Work out the finished part from the listing and answer in its coordinate system (mm). A direction names the side the tool comes from. Coordinates: 2 decimals unless noted, no trailing zeros. Loops run counter-clockwise (first coordinate to the right, second up) from the corner with the lowest first, then second, coordinate; pieces in that order, holes last. Notation, with made-up numbers: (18.25, 49) -> (46.25, 49) arc R38 ccw to (46.25, 88) -> close; hole circle Ø1 at (27, 20.5). An arc over 180 degrees is marked (long way). Use a Markdown table: item, result.
from build123d import *

# Parameters (mm, degrees)
SKETCH2_W           = 25
SKETCH2_H           = 25
BOSS_EXTRUDE1_DEPTH = 25
SKETCH3_R           = 3.25
CUT_EXTRUDE1_DEPTH  = 44.301270189
SKETCH4_R           = 3.25
CUT_EXTRUDE2_DEPTH  = 44.301270189
SKETCH5_R           = 3.25
CUT_EXTRUDE3_DEPTH  = 44.301270189
SKETCH6_R           = 5
CUT_EXTRUDE4_DEPTH  = 23
SKETCH7_R           = 5
CUT_EXTRUDE5_DEPTH  = 23
SKETCH12_R          = 5
CUT_EXTRUDE9_DEPTH  = 23
BOSS_EXTRUDE2_DEPTH = 1
BOSS_EXTRUDE3_DEPTH = 1
BOSS_EXTRUDE4_DEPTH = 1
FILLET2_R           = 3


with BuildPart() as part:
    # Sketch2 → Boss-Extrude1 (new body)
    with BuildSketch(Plane(origin=(0, 0, 0), x_dir=(1, 0, 0), z_dir=(0, 1, 0))):
        with Locations((12.5, 12.5)):
            Rectangle(SKETCH2_W, SKETCH2_H)
    extrude(amount=BOSS_EXTRUDE1_DEPTH)

    # Sketch3 → Cut-Extrude1 (cut, through all)
    with BuildSketch(Plane(origin=(0, 25, 0), x_dir=(1, 0, 0), z_dir=(0, 1, 0))):
        with Locations(Location((10, 10, 0), (0, 0, 270))):
            Circle(SKETCH3_R)
    extrude(amount=-CUT_EXTRUDE1_DEPTH, mode=Mode.SUBTRACT)

    # Sketch4 → Cut-Extrude2 (cut, through all)
    with BuildSketch(Plane.ZY):
        with Locations((-10, 15)):
            Circle(SKETCH4_R)
    extrude(amount=-CUT_EXTRUDE2_DEPTH, mode=Mode.SUBTRACT)

    # Sketch5 → Cut-Extrude3 (cut, through all)
    with BuildSketch(Plane.XY):
        with Locations((10, 15)):
            Circle(SKETCH5_R)
    extrude(amount=-CUT_EXTRUDE3_DEPTH, mode=Mode.SUBTRACT)

    # Sketch6 → Cut-Extrude4 (cut)
    with BuildSketch(Plane(origin=(0, 0, -25), x_dir=(-1, 0, 0), z_dir=(0, 0, -1))):
        with Locations((-10, 15)):
            Circle(SKETCH6_R)
    extrude(amount=-CUT_EXTRUDE4_DEPTH, mode=Mode.SUBTRACT)

    # Sketch7 → Cut-Extrude5 (cut)
    with BuildSketch(Plane(origin=(25, 0, 0), x_dir=(0, 0, -1), z_dir=(1, 0, 0))):
        with Locations((10, 15)):
            Circle(SKETCH7_R)
    extrude(amount=-CUT_EXTRUDE5_DEPTH, mode=Mode.SUBTRACT)

    # Sketch12 → Cut-Extrude9 (cut)
    with BuildSketch(Plane.XZ):
        with Locations(Location((10, -10, 0), (0, 0, 270))):
            Circle(SKETCH12_R)
    extrude(amount=-CUT_EXTRUDE9_DEPTH, mode=Mode.SUBTRACT)

    # Sketch19 → Boss-Extrude2 (add)
    with BuildSketch(Plane.XY):
        Polygon((20, 25), (20, 5), (0, 5), (0, 0), (25, 0), (25, 25), align=None)
    extrude(amount=BOSS_EXTRUDE2_DEPTH)

    # Sketch20 → Boss-Extrude3 (add)
    with BuildSketch(Plane(origin=(0, 25, 0), x_dir=(1, 0, 0), z_dir=(0, 1, 0))):
        Polygon((20, 0), (20, 20), (0, 20), (0, 25), (25, 25), (25, -1), (20, -1), align=None)
    extrude(amount=BOSS_EXTRUDE3_DEPTH)

    # Sketch21 → Boss-Extrude4 (add)
    with BuildSketch(Plane.ZY):
        Polygon((-20, 5), (0, 5), (1, 5), (1, 0), (-25, 0), (-25, 26), (-20, 26), (-20, 25), align=None)
    extrude(amount=BOSS_EXTRUDE4_DEPTH)

    # Fillet2
    fillet2_edges = [part.edges().sort_by_distance(p)[0] for p in [
        (12, 0, 1),
        (25, 13, 1),
        (25, 26, -12),
        (12, 26, -25),
        (-1, 13, -25),
        (-1, 0, -12),
        (12, 0, -25),
        (25, 0, -12),
        (25, 13, -25),
    ]]
    fillet(fillet2_edges, radius=FILLET2_R)


solid = part.part
Q1. Given pin 1 Ø6.5 at (y, z) = (16.5, -10.5) entering from -X; pin 2 Ø5 at (x, y) = (9, 15) entering from -Z; pin 3 Ø3 at (x, z) = (8, -8) entering from -Y, each flat-ended and moving along its own axis, determine where each tip first touches the part or whether it passes through.
Solved:
| item | result |
|---|---|
| pin 1 | x = 0 |
| pin 2 | z = -2 |
| pin 3 | y = 23 |
Q2. Section A-A on z = -10 is taken. State how many separate pieces and enclosed holes the cut face has, and give its area (3 significant figures).
Solved:
| item | result |
|---|---|
| separate pieces | 4 |
| enclosed holes | 0 |
| area | 243 mm² |
Q3. Determine the mould class of faces 1 (the flat face through (9, 23, -13.3)), 2 (the cylindrical face through (24.14, 25.1, -10.34)), 3 (the cylindrical face through (4, 18, -6)) for opening direction Y: pulls with the +Y half, pulls with the -Y half, needs draft (parallel to the pull), parting line crosses it, or undercut.
Solved:
| item | result |
|---|---|
| face 1 | pulls with the -Y half |
| face 2 | pulls with the +Y half |
| face 3 | undercut |
Q4. For faces 4 (the cylindrical face through (14, 18, -19)), 5 (the cylindrical face through (13, 21, -6)), 6 (the flat face through (10, 10, 0)), 7 (the cylindrical face through (19, 18, -6)), determine the directions among +Z, -Z, +X, -X, +Y, -Y from which every point of the face is accessible in a straight line to the end or side of a thin tool.
Solved:
| item | result |
|---|---|
| face 4 | -Z |
| face 5 | -Y |
| face 6 | +Z, -X, +Y |
| face 7 | +X |
Q5. Section C-C on y = 6.25 is taken. Determine the outline of the cut face in (x, z), and give its area (3 significant figures).
Solved:
| item | result |
|---|---|
| outline | (-1, -22) arc R3 ccw to (2, -25) -> (22, -25) arc R3 ccw to (25, -22) -> (25, -2) arc R3 ccw to (22, 1) -> (20, 1) -> (20, 0) -> (0, 0) -> (0, -20) -> (-1, -20) -> close; hole circle Ø10 at (10, -10) |
| area | 551 mm² |
Q6. Consider line 1 (Y direction, x = 4.15, z = -10); line 2 (Z direction, x = 3.7, y = 15); line 3 (Z direction, x = 10, y = 3). Determine where each line is inside the solid, lowest interval first. Write a range as [from, to].
Solved:
| item | result |
|---|---|
| line 1 | [0, 10], [20, 25] |
| line 2 | [-25, -15], [-5, 0] |
| line 3 | [-25, -15], [-5, 1] |
Q7. Section D-D on x = 2.75 is taken. Determine the outline of the cut face in (y, z).
Solved:
| item | result |
|---|---|
| outline | (0, -22) arc R3 ccw to (3, -25) -> (23, -25) arc R3 ccw to (26, -22) -> (26, -20) -> (25, -20) -> (25, 0) -> (5, 0) -> (5, 1) -> (3, 1) arc R3 ccw to (0, -2) -> close; hole circle Ø10 at (15, -10) |
